The figure shows three views and two pictorial views of one solid part (mm, origin at its lowest corner). Answer the questions. A direction names the side the tool comes from. Coordinates: 2 decimals unless noted, no trailing zeros. Write each loop counter-clockwise with the first axis right and the second up, starting at its lowest first coordinate (ties: lowest second). Pieces come first, ordered by that corner, then holes.
Item 1: Section A-A (z = 4) is taken. Give the vertices of the cut face in (x, y) (1 decimal).
Item 2: Section C-C (x = 5) is taken. Give the vertices of the cut face in (y, z).
Item 3: Determine the mould class of the marked faces 1, 2, 3 and 4 for opening direction X: released by +X, released by -X, zero draft, split by the parting line, or undercut.
Item 4: Section D-D (z = 16) is taken. Give the vertices of the cut face in (x, y).
Item 5: Straight lines are drawn through the part: probe 1 along Z at (x, y) = (13, 16.25); probe 2 along X at (y, z) = (24.25, 5) (1 decimal); probe 3 along X at (y, z) = (21.25, 27.5) (1 decimal). For each, find the intervals that lie inside material, in ascending order.
Item 6: Each of these flat-tipped pins is pushed along its axis until it touches: P1, Ø1, axis at x = 10, z = 28, coming from the -Y side; P2, Ø1, axis at y = 19.5, z = 11.5, coming from the +X side; P3, Ø1, axis at y = 13.5, z = 28, coming from the -X side (1 decimal); P4, Ø5, axis at y = 10, z = 4, coming from the +X side. Where does it stop, or does it pass through?
Item 7: A tool of negligible diameter and unlimited length cuts with its end or side. For the marked faces 5 and 6, from which of +Z, -Z, +X, -X, +Y, -Y can it reach the whole face along a straight path? Write none if from no direction.
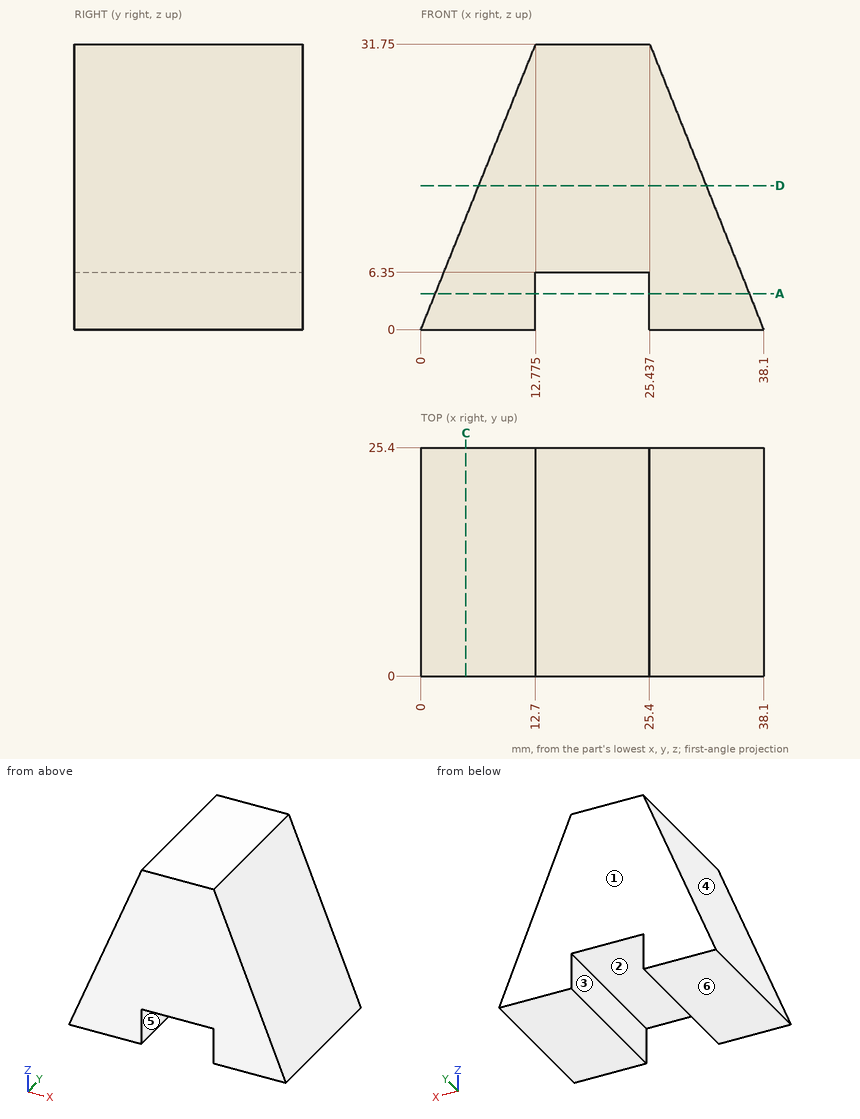
Established:
1. outline: (1.6, 0) - (12.7, 0) - (12.7, 25.4) - (1.6, 25.4) - close; (25.4, 0) - (36.5, 0) - (36.5, 25.4) - (25.4, 25.4) - close
2. outline: (0, 0) - (25.4, 0) - (25.4, 12.43) - (0, 12.43) - close
3. face 1: zero draft
3. face 2: undercut
3. face 3: undercut
3. face 4: released by -X
4. outline: (6.44, 0) - (31.72, 0) - (31.72, 25.4) - (6.44, 25.4) - close
5. probe 1: z = 6.35 to 31.75
5. probe 2: x = 2 to 12.7, 25.4 to 36.1
5. probe 3: x = 11.1 to 27.1
6. P1: passes through
6. P2: stops at x = 33.71
6. P3: stops at x = 11.1
6. P4: stops at x = 37.5
7. face 5: -Z, +Y, -Y
7. face 6: -Z, +X, -X, +Y, -Y
